```python
from build123d import *

# Parameters (mm, degrees)
F0_W          = 125.3066509962
F0_H          = 116.8914437294
F2_DEPTH      = 25.4
F3_DEPTH      = 54.8134744167
F4_R          = 19.141083189
F4_R_2        = 14.402572036
F5_DEPTH      = 65.8841822296
F7_W          = 17.8398638964
F7_H          = 29.3952524662
F8_DEPTH      = 25.4
F8_DEPTH_BACK = 25.4


# Not quite as in the source:
# - a fillet or chamfer that OpenCascade refuses, or shapes differently, is made with other operations: its cross-section is extruded or revolved along the edge and cut away or added


with BuildPart() as f2:
    # F0 (on Front) → F2 (new body)
    with BuildSketch(Plane.XZ):
        Rectangle(F0_W, F0_H)
    extrude(amount=F2_DEPTH)

    # F1 (on face) → F3 (join)
    with BuildSketch(Plane.XZ):
        with BuildLine():
            ThreePointArc((34.7187500455, -33.271908015), (44.6203470202, -17.9286390861), (48.0875396302, 0))
            ThreePointArc((48.0875396302, 0), (47.9767259565, 3.262703507), (47.6447956571, 6.5103697647))
            ThreePointArc((47.6447956571, 6.5103697647), (37.5878279083, 12.213025626), (42.3721487148, 22.7379084564))
            ThreePointArc((42.3721487148, 22.7379084564), (28.2651466136, 38.9036367785), (8.5313219634, 47.3247082742))
            ThreePointArc((8.5313219634, 47.3247082742), (0, 39.5221811368), (-8.5313219634, 47.3247082742))
            ThreePointArc((-8.5313219634, 47.3247082742), (-28.2651466136, 38.9036367785), (-42.3721487148, 22.7379084564))
            ThreePointArc((-42.3721487148, 22.7379084564), (-38.5869212276, 19.5805755678), (-37.1686094245, 14.8598669634))
            ThreePointArc((-37.1686094245, 14.8598669634), (-40.3955017751, 8.1616473967), (-47.6447956571, 6.5103697647))
            ThreePointArc((-47.6447956571, 6.5103697647), (-45.7339679179, -14.8598669634), (-34.7187500455, -33.271908015))
            ThreePointArc((-34.7187500455, -33.271908015), (-25.2578272797, -30.88357465), (-19.6997881202, -38.9036367785))
            ThreePointArc((-19.6997881202, -38.9036367785), (-20.0091221024, -41.1847385714), (-20.9147811398, -43.3010784803))
            ThreePointArc((-20.9147811398, -43.3010784803), (0, -48.0875396302), (20.9147811398, -43.3010784803))
            ThreePointArc((20.9147811398, -43.3010784803), (23.2305552106, -31.9741161944), (34.7187500455, -33.271908015))
        make_face()
    extrude(amount=-F3_DEPTH)

    # F4 (on face) → F5 (join)
    with BuildSketch(Plane(origin=(0, 54.8134744167, 0), x_dir=(-1, 0, 0), z_dir=(0, 1, 0))):
        Circle(F4_R)
        Circle(F4_R_2, mode=Mode.SUBTRACT)
    extrude(amount=F5_DEPTH)

    # F6: fillet of radius 16.8234648582 on 1 edges, made by hand

    # F6_s1 → F6_t2 (revolve, cut)
    with BuildSketch(Plane.XY):
        with BuildLine():
            ThreePointArc((-19.141083189, 108.9936887817), (-17.9115236115, 115.3070941964), (-14.402572036, 120.6976566464))
            Line((-14.402572036, 120.6976566464), (-19.141083189, 120.6976566464))
            Line((-19.141083189, 120.6976566464), (-19.141083189, 108.9936887817))
        make_face()
    revolve(axis=Axis((0, 120.6976566464, 0), (0, 1, 0)), mode=Mode.SUBTRACT)

    # F7 (on Right) → F8 (cut, two sides)
    with BuildSketch(Plane.YZ) as f8_sk:
        with Locations((85.9047025442, 0)):
            Rectangle(F7_W, F7_H)
    extrude(amount=-F8_DEPTH, mode=Mode.SUBTRACT)
    extrude(f8_sk.sketch, amount=F8_DEPTH_BACK, mode=Mode.SUBTRACT)


solid = f2.part
```
Verification items for the finished model (mm, model axes). A direction names the side the tool comes from. Coordinates: 2 decimals unless noted, no trailing zeros. Order: outer loops, then holes, each group sorted by start corner. A loop starts at its lowest first (then second) coordinate and runs counter-clockwise, first axis right, second up. Notation, with made-up numbers: (-18.75, -6) - (14.25, -6) arc R33 cw to (14.25, 28) - close; hole circle Ø11 at (-2.75, 54.5). An arc over 180 degrees is marked (long way). Return JSON: item names as keys, results as strings.
(1) Mould release check, pull along Y, two halves, no side actions. Record for faces 1 (the flat face through (-1, 54.813, 21)), 2 (the cylindrical face through (37.644, 27.023, 12.045)), 3 (the flat face through (-14, 76.985, -4)): pulls with the +Y half, pulls with the -Y half, needs draft (parallel to the pull), parting line crosses it, or undercut.
Filled sheet:
{"face 1": "pulls with the +Y half", "face 2": "needs draft", "face 3": "undercut"}
(2) Section check B-B, the plane y = 70.5. Record the cut outline in (x, z).
Filled sheet:
{"outline": "circle Ø38.28 at (0, 0); hole circle Ø28.81 at (0, 0)"}
(3) Section check A-A, the plane y = 11. Record the cut outline in (x, z).
Filled sheet:
{"outline": "(-47.64, 6.51) arc R48.09 ccw to (-34.72, -33.27) arc R8.57 cw to (-20.91, -43.3) arc R48.09 ccw to (20.91, -43.3) arc R8.57 cw to (34.72, -33.27) arc R48.09 ccw to (47.64, 6.51) arc R8.57 cw to (42.37, 22.74) arc R48.09 ccw to (8.53, 47.32) arc R8.57 cw to (-8.53, 47.32) arc R48.09 ccw to (-42.37, 22.74) arc R8.57 cw to start"}
(4) Section check D-D, the plane x = -30.5. Record the cut outline in (y, z), and give its area (3 significant figures).
Filled sheet:
{"outline": "(-25.4, -58.45) - (0, -58.45) - (0, -30.63) - (54.81, -30.63) - (54.81, 37.18) - (0, 37.18) - (0, 58.45) - (-25.4, 58.45) - close", "area": "6,690 mm^2"}
(5) Access from +Z, -Z, +X, -X, +Y, -Y to the whole of each face (thin tool, end or side, straight path). Record for faces 4 (the flat face through (0, 86, 14.698)), 5 (the cylindrical face through (-0.303, 27.023, -48.087)), 6 (the cylindrical face through (14.39, 107.58, 0.63)), 7 (the cylindrical face through (0.178, 27.023, 39.524)).
Filled sheet:
{"face 4": "+X, -X", "face 5": "-Z, +Y", "face 6": "+Y", "face 7": "+Z, +Y"}
(6) Go/stop test with flat-tipped pins: pin 1 (14.5 mm diameter, centred on x = -0.5, y = 84.5, fed in from +Z); pin 2 (6 mm diameter, centred on y = 5.5, z = -12, fed in from +X); pin 3 (9 mm diameter, centred on x = 5.5, z = 4, fed in from +Y). Record where each tip stops, or that it passes through.
Filled sheet:
{"pin 1": "stops at z = 19.14", "pin 2": "stops at x = 47.24", "pin 3": "stops at y = 54.81"}
(7) Thickness scan on line 1 along X through (y, z) = (63, 0); line 2 along Y through (x, z) = (27, 38.5). Record the ranges inside material, lowest first.
Filled sheet:
{"line 1": "x = -19.14 to -14.4, 14.4 to 19.14", "line 2": "y = -25.4 to 54.81"}
(8) Section check C-C, the plane z = 26. Record the cut outline in (x, y), and give its area (3 significant figures).
Filled sheet:
{"outline": "(-62.65, -25.4) - (62.65, -25.4) - (62.65, 0) - (40.45, 0) - (40.45, 54.81) - (-40.45, 54.81) - (-40.45, 0) - (-62.65, 0) - close", "area": "7,620 mm^2"}
